```python
from build123d import *

# Parameters (mm, degrees)
SKETCH1_R           = 9
BOSS_EXTRUDE1_DEPTH = 6.5
SKETCH2_R           = 9
SKETCH2_R_2         = 6
CUT_EXTRUDE2_DEPTH  = 5
SKETCH3_R           = 2.75
CUT_EXTRUDE3_DEPTH  = 19.193405399


with BuildPart() as part:
    # Sketch1 → Boss-Extrude1 (new, symmetric)
    with BuildSketch(Plane.XY):
        with Locations(Location((0, 0, 0), (0, 0, 180))):
            Circle(SKETCH1_R)
    extrude(amount=BOSS_EXTRUDE1_DEPTH, both=True)

    # Sketch2 → Cut-Extrude2 (cut, symmetric)
    with BuildSketch(Plane.XY):
        with Locations(Location((0, 0, 0), (0, 0, 180))):
            Circle(SKETCH2_R)
        Circle(SKETCH2_R_2, mode=Mode.SUBTRACT)
    extrude(amount=CUT_EXTRUDE2_DEPTH, both=True, mode=Mode.SUBTRACT)

    # Sketch3 → Cut-Extrude3 (cut, through all)
    with BuildSketch(Plane.XY.offset(6.5)):
        Circle(SKETCH3_R)
    extrude(amount=-CUT_EXTRUDE3_DEPTH, mode=Mode.SUBTRACT)


solid = part.part
```
Geometry: final body of the model. Coordinates: model frame, mm. A direction names the side the tool comes from. Round coordinates to 2 decimals unless told otherwise and drop trailing zeros. Order: outer loops, then holes, each group sorted by start corner. A loop starts at its lowest first (then second) coordinate and runs counter-clockwise, first axis right, second up. Notation, with made-up numbers: (-27, 66) -> (20, 66) arc R8 cw to (20, 75) -> close; hole circle Ø11 at (-39.75, 55.5). An arc over 180 degrees is marked (long way). Use one line per item in the form item = value. Start each with the question number.
1. Cut plane C-C (z = -0.5). Return the cut outline in (x, y).
2. Draft query along Z for faces 1 (the face through (6.633, -6.083, 5.76)), 2 (the face through (-2, 6, -5)), 3 (the face through (2.1, -2.1, -6.5)). Return one class per face: pulls with the +Z half, pulls with the -Z half, needs draft (parallel to the pull), parting line crosses it, or undercut.
3. Cut plane D-D (y = 4.5). Return the cut outline in (x, z).
4. Line query: probe 1 along Z at (x, y) = (-5.5, -5.75); probe 2 along Y at (x, z) = (0, -2.5); probe 3 along Y at (x, z) = (1.25, -0.5). Output: solid intervals per line, ascending.
5. Cut plane A-A (y = 0). Return the cut outline in (x, z).
6. Reachability of faces 4 (the face through (-2, 6, 5)), 5 (the face through (2.1, -2.1, 6.5)) from +Z, -Z, +X, -X, +Y, -Y: full face, straight path, thin tool, end or side. Return the list, or none.
7. Pin query (flat end, axial travel): pin 1 Ø2 at (x, z) = (-5, -0.5) entering from +Y; pin 2 Ø2 at (x, z) = (3, -2.5) entering from -Y; pin 3 Ø2 at (x, z) = (-7, 5) entering from -Y. Return the tip coordinate at first contact, or that it passes through.
Solution:
q1.outline = circle Ø12 at (0, 0); hole circle Ø5.5 at (0, 0)
q2.face_1 = needs draft
q2.face_2 = undercut
q2.face_3 = pulls with the -Z half
q3.outline = (-7.79, -6.5) -> (7.79, -6.5) -> (7.79, -5) -> (3.97, -5) -> (3.97, 5) -> (7.79, 5) -> (7.79, 6.5) -> (-7.79, 6.5) -> (-7.79, 5) -> (-3.97, 5) -> (-3.97, -5) -> (-7.79, -5) -> close
q4.probe_1 = -6.5 to -5, 5 to 6.5
q4.probe_2 = -6 to -2.75, 2.75 to 6
q4.probe_3 = -5.87 to -2.45, 2.45 to 5.87
q5.outline = (-9, -6.5) -> (-2.75, -6.5) -> (-2.75, 6.5) -> (-9, 6.5) -> (-9, 5) -> (-6, 5) -> (-6, -5) -> (-9, -5) -> close; (2.75, -6.5) -> (9, -6.5) -> (9, -5) -> (6, -5) -> (6, 5) -> (9, 5) -> (9, 6.5) -> (2.75, 6.5) -> close
q6.face_4 = none
q6.face_5 = +Z, +X, -X, +Y, -Y
q7.pin_1 = 4.47
q7.pin_2 = -5.66
q7.pin_3 = -6.71
